Source: CAD feature listing. Evaluate the final solid. Frame: model axes, mm. Give positions to 0.01 mm unless a question says otherwise; leave off trailing zeros. Loops run counter-clockwise (first coordinate to the right, second up) from the corner with the lowest first, then second, coordinate; pieces in that order, holes last.
```python
from build123d import *

# Parameters (mm, degrees)
CROQUIS1_R              = 5
SALIENTE_EXTRUIR1_DEPTH = 5


with BuildPart() as part:
    # Croquis1 → Saliente-Extruir1 (new body)
    with BuildSketch(Plane(origin=(0, 0, 0), x_dir=(0, 0, -1), z_dir=(1, 0, 0))):
        with BuildLine():
            Line((188, -5), (12, -5))
            ThreePointArc((12, -5), (-13, 0), (12, 5))
            Line((12, 5), (188, 5))
            ThreePointArc((188, 5), (213, 0), (188, -5))
        make_face()
        with Locations((200, 0)):
            Circle(CROQUIS1_R, mode=Mode.SUBTRACT)
        with BuildLine():
            Line((-2, 0), (-2, 2.236067977))
            ThreePointArc((-2, 2.236067977), (3, 0), (-2, -2.236067977))
            Line((-2, -2.236067977), (-2, 0))
        make_face(mode=Mode.SUBTRACT)
    extrude(amount=SALIENTE_EXTRUIR1_DEPTH)


solid = part.part
```
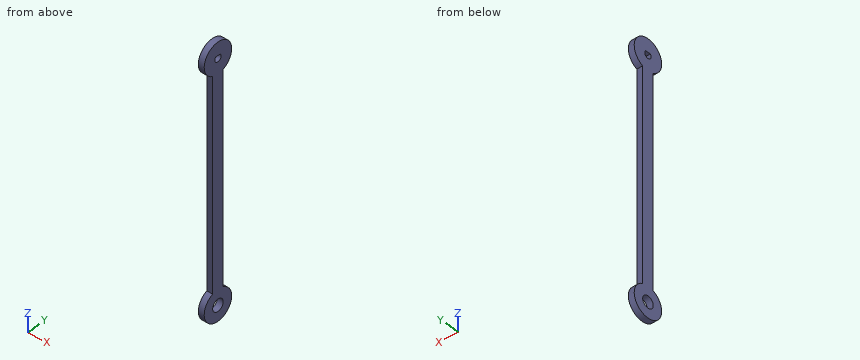
(1) Ray query, line 1 along Y through (x, z) = (2.2, -200); line 2 along Y through (x, z) = (1.8, 0); line 3 along Y through (x, z) = (3.6, -26). Return the intervals inside material, ascending.
A:
line 1: y = -13 to -5, 5 to 13
line 2: y = -13 to -3, 3 to 13
line 3: y = -5 to 5
(2) Section D-D, the plane z = -200. Return the cut outline in (x, y).
A:
outline: (0, -13) - (5, -13) - (5, -5) - (0, -5) - close; (0, 5) - (5, 5) - (5, 13) - (0, 13) - close
(3) Section A-A, the plane z = 0. Return the cut outline in (x, y), then the cut area to 3 significant figures.
A:
outline: (0, -13) - (5, -13) - (5, -3) - (0, -3) - close; (0, 3) - (5, 3) - (5, 13) - (0, 13) - close
area: 100 mm2
(4) Section C-C, the plane x = 3.45. Return the cut outline in (y, z).
A:
outline: (-5, -188) arc R13 ccw (long way) to (5, -188) - (5, -12) arc R13 ccw (long way) to (-5, -12) - close; hole circle Ø10 at (0, -200); hole (-2.24, 2) arc R3 ccw (long way) to (2.24, 2) - close
(5) First-contact query: pin 1 (2.5 mm diameter, centred on x = 3, z = -129.5, fed in from -Y); pin 2 (6 mm diameter, centred on y = 0, z = -200, fed in from +X); pin 3 (1.5 mm diameter, centred on x = 1.5, z = -116.5, fed in from +Y). Flat tips, straight axial feed; report the tip coordinate or a pass-through.
A:
pin 1: stops at y = -5
pin 2: passes through
pin 3: stops at y = 5
(6) Section B-B, the plane y = 0. Return the cut outline in (x, z).
A:
outline: (0, -213) - (5, -213) - (5, -205) - (0, -205) - close; (0, -195) - (5, -195) - (5, -3) - (0, -3) - close; (0, 2) - (5, 2) - (5, 13) - (0, 13) - close
